from build123d import *

# Parameters (mm, degrees)
F0_W     = 76.2
F0_H     = 76.2
F1_DEPTH = 152.4
F2_DEPTH = 152.4
F3_W     = 76.2
F3_H     = 76.2
F4_DEPTH = 203.2
F5_W     = 1209.04
F5_H     = 76.2
F6_DEPTH = 711.2


with BuildPart() as f1:
    # F0 (on Top) → F1 (new body)
    with BuildSketch(Plane.XY):
        with Locations((38.1, 38.1)):
            Rectangle(F0_W, F0_H)
    extrude(amount=F1_DEPTH)



with BuildPart() as f2:
    # F0 (on Top) → F2 (new body)
    with BuildSketch(Plane.XY):
        with Locations((38.1, 520.7)):
            Rectangle(F0_W, F0_H)
    extrude(amount=F2_DEPTH)


with BuildPart() as f2b:
    # F0 (on Top) → F2, piece 2 (new body)
    with BuildSketch(Plane.XY):
        with Locations((1460.5, 520.7)):
            Rectangle(F0_W, F0_H)
    extrude(amount=F2_DEPTH)


with BuildPart() as f2c:
    # F0 (on Top) → F2, piece 3 (new body)
    with BuildSketch(Plane.XY):
        with Locations((1460.5, 38.1)):
            Rectangle(F0_W, F0_H)
    extrude(amount=F2_DEPTH)


with BuildPart() as f1_1:
    add(f1.part)

    add(f2.part)  # F4 merges F2

    add(f2b.part)  # F4 merges F2b

    add(f2c.part)  # F4 merges F2c
    # F3 (on face) → F4 (join)
    with BuildSketch(Plane.XY.offset(152.4)):
        Polygon((76.2, 76.2), (76.2, 0), (1498.6, 0), (1498.6, 558.8), (0, 558.8), (0, 76.2), align=None)
        with Locations((38.1, 38.1)):
            Rectangle(F3_W, F3_H)
    extrude(amount=F4_DEPTH)

    # F5 (on face) → F6 (join)
    with BuildSketch(Plane.XY.offset(355.6)):
        with Locations((749.3, 215.9)):
            Rectangle(F5_W, F5_H)
    extrude(amount=F6_DEPTH)


solid = f1_1.part
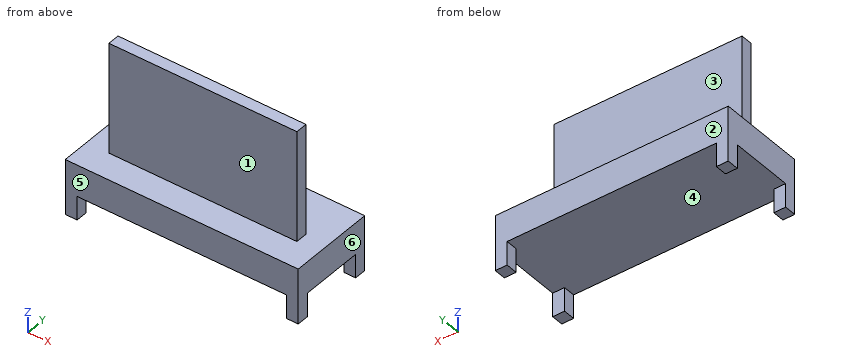
Source: CAD feature listing. Evaluate the final solid. Frame: model axes, mm. Face numbers are marked on the shaded views. A direction names the side the tool comes from. Round coordinates to 2 decimals unless told otherwise and drop trailing zeros. Loops run counter-clockwise (first coordinate to the right, second up) from the corner with the lowest first, then second, coordinate; pieces in that order, holes last. Notation, with made-up numbers: (-11.75, 27.5) - (-4.75, 27.5) arc R36 ccw to (-4.75, 63.5) - close; hole circle Ø8 at (16.25, -9). An arc over 180 degrees is marked (long way). Write item = value, one per line. Start each with the question number.
(1) Section query D-D, the plane y = 105. Output: boundary loops of the cut face in (x, z).
(2) Pull-direction query (X, two-part tool) for the marked faces 4, 5 and 6; classes: +X half, -X half, draft (parallel to the pull), parting line (faces both ways), or undercut.
(3) Set-up query: the marked faces 1, 2 and 3. Return all of +Z, -Z, +X, -X, +Y, -Y with unobstructed straight access to the full face (end or side cutting, diameter ignored); none if empty.
(4) Section query A-A, the plane y = 235. Output: boundary loops of the cut face in (x, z).
(5) Section query B-B, the plane x = 1050. Output: boundary loops of the cut face in (y, z), plus the area to 3 significant figures.
(6) Ray query, line 1 along Y through (x, z) = (443.5, 984.5); line 2 along Z through (x, y) = (212, 117.5); line 3 along X through (y, z) = (244.5, 932.5). Return the intervals inside material, ascending. Write a range as from..to.
(7) Pin query (flat end, axial travel): pin 1 (6 mm diameter, centred on x = 901, z = 424.5, fed in from -Y); pin 2 (1.5 mm diameter, centred on x = 1030, y = 314.5, fed in from +Z); pin 3 (23 mm diameter, centred on y = 198.5, z = 575, fed in from -X). Return the tip coordinate at first contact, or that it passes through.
(8) Section query C-C, the plane z = 394.5. Output: boundary loops of the cut face in (x, y), plus the area to 3 significant figures.
Conclusion:
q1.outline = (0, 152.4) - (1498.6, 152.4) - (1498.6, 355.6) - (0, 355.6) - close
q2.face_4 = undercut
q2.face_5 = draft
q2.face_6 = +X half
q3.face_1 = +Z, +X, -X, -Y
q3.face_2 = +Z, -Z, +X, -X, +Y
q3.face_3 = +Z, +X, -X, +Y
q4.outline = (0, 152.4) - (1498.6, 152.4) - (1498.6, 355.6) - (1353.82, 355.6) - (1353.82, 1066.8) - (144.78, 1066.8) - (144.78, 355.6) - (0, 355.6) - close
q5.outline = (0, 152.4) - (558.8, 152.4) - (558.8, 355.6) - (254, 355.6) - (254, 1066.8) - (177.8, 1066.8) - (177.8, 355.6) - (0, 355.6) - close
q5.area = 168,000 mm2
q6.line_1 = 177.8..254
q6.line_2 = 152.4..355.6
q6.line_3 = 144.78..1353.82
q7.pin_1 = 177.8
q7.pin_2 = 355.6
q7.pin_3 = 144.78
q8.outline = (144.78, 177.8) - (1353.82, 177.8) - (1353.82, 254) - (144.78, 254) - close
q8.area = 92,100 mm2
